```python
from build123d import *

# Parameters (mm, degrees)
F1_DEPTH = 304.8
F0_W     = 38.1
F0_H     = 127
F2_DEPTH = 304.8
F3_W     = 38.1
F3_H     = 12.7
F4_DEPTH = 165.101


with BuildPart() as f1:
    # F0 (on Front) → F1 (new body)
    with BuildSketch(Plane.XZ):
        Polygon((51.189408, 97.00968), (-88.510592, 97.00968), (-88.510592, 58.90968), (-88.510592, -68.09032), (-88.510592, -106.19032), (51.189408, -106.19032), align=None)
    extrude(amount=F1_DEPTH)

    # F0 (on Front) → F2 (join)
    with BuildSketch(Plane.XZ):
        with Locations((-107.560592, -4.59032)):
            Rectangle(F0_W, F0_H)
    extrude(amount=F2_DEPTH)

    # F3 (on face) → F4 (cut, through all)
    with BuildSketch(Plane.XY.offset(58.90968)):
        with Locations((-107.560592, -6.35)):
            Rectangle(F3_W, F3_H)
        Polygon((-88.510592, -304.8), (-126.610592, -266.7), (-126.610592, -304.8), align=None)
    extrude(amount=-F4_DEPTH, mode=Mode.SUBTRACT)


solid = f1.part
```
Source: CAD feature listing. Evaluate the final solid. Frame: model axes, mm. A direction names the side the tool comes from. Coordinates: 2 decimals unless noted, no trailing zeros. Loops run counter-clockwise (first coordinate to the right, second up) from the corner with the lowest first, then second, coordinate; pieces in that order, holes last. Notation, with made-up numbers: (70.5, -23.5) - (98.5, -23.5) arc R15 ccw to (98.5, -14.5) - close; hole circle Ø5 at (-34.5, 38.25). An arc over 180 degrees is marked (long way). Answer as CSV lines item,"result".
1. Section C-C (z = 73). Return loops of the section in (x, y).
Established:
outline,"(-88.51, -304.8) - (51.19, -304.8) - (51.19, 0) - (-88.51, 0) - close"
2. Section D-D (x = -94.5). Return loops of the section in (y, z), then the cut area to 3 significant figures.
Established:
outline,"(-298.81, -68.09) - (-12.7, -68.09) - (-12.7, 58.91) - (-298.81, 58.91) - close"
area,"36,300 mm2"
3. Section A-A (z = -3.5). Return loops of the section in (x, y).
Established:
outline,"(-126.61, -266.7) - (-88.51, -304.8) - (51.19, -304.8) - (51.19, 0) - (-88.51, 0) - (-88.51, -12.7) - (-126.61, -12.7) - close"
4. Ray query, line 1 (X direction, y = -256.5, z = 67); line 2 (X direction, y = -280, z = 1); line 3 (Y direction, x = -89.5, z = 27.5). Return the intervals inside material, ascending.
Established:
line 1,"x = -88.51 to 51.19"
line 2,"x = -113.31 to 51.19"
line 3,"y = -303.81 to -12.7"
5. Contact query for flat-ended pins moving along their axis: pin 1 (3 mm diameter, centred on x = -90.5, y = -120.5, fed in from +Z); pin 2 (3 mm diameter, centred on y = -52.5, z = 64, fed in from -X). Output: stop coordinate, or through.
Established:
pin 1,"stops at z = 58.91"
pin 2,"stops at x = -88.51"
6. Reachability of faces 1 (the flat face through (51.189, -150, -6)), 2 (the flat face through (-108, -12.7, -4)), 3 (the flat face through (-20, 0, -3)), 4 (the flat face through (-108, -157, -68.09)), 5 (the flat face through (-108, -157, 58.91)) from +Z, -Z, +X, -X, +Y, -Y: full face, straight path, thin tool, end or side. Return the list, or none.
Established:
face 1,"+Z, -Z, +X, +Y, -Y"
face 2,"+Z, -Z, -X, +Y"
face 3,"+Z, -Z, +X, -X, +Y"
face 4,"-Z, -X, +Y, -Y"
face 5,"+Z, -X, +Y, -Y"
7. Section B-B (y = -223). Return loops of the section in (x, z).
Established:
outline,"(-126.61, -68.09) - (-88.51, -68.09) - (-88.51, -106.19) - (51.19, -106.19) - (51.19, 97.01) - (-88.51, 97.01) - (-88.51, 58.91) - (-126.61, 58.91) - close"
